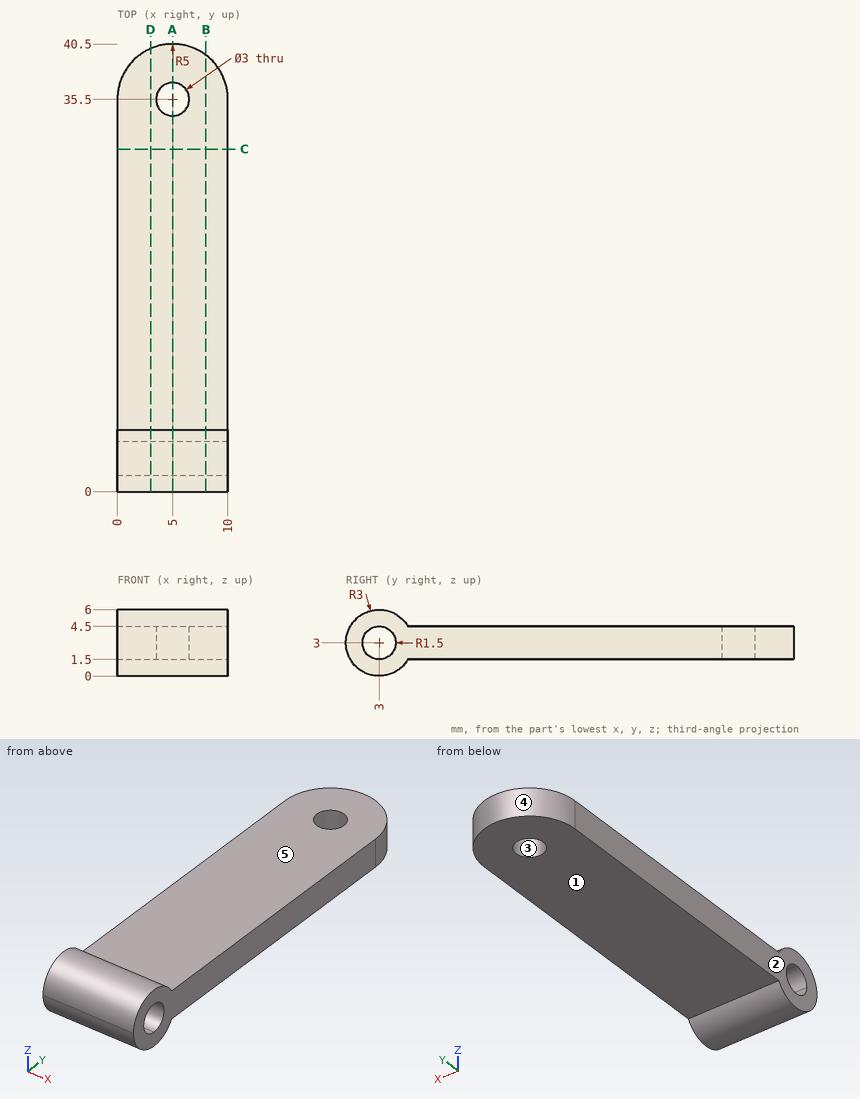
Geometry check sheet. Reference: drawing and pictorial views, mm from the part's lowest x, y, z. A direction names the side the tool comes from. Coordinates: 2 decimals unless noted, no trailing zeros. Write each loop counter-clockwise with the first axis right and the second up, starting at its lowest first coordinate (ties: lowest second). Pieces come first, ordered by that corner, then holes. Notation, with made-up numbers: (61.5, 34.25) -> (88.5, 34.25) arc R24 cw to (88.5, 66.25) -> close; hole circle Ø5 at (28, 37). An arc over 180 degrees is marked (long way). Use a Markdown table: item, result.
1. Tool access check on the marked faces 1 and 2. Record the directions out of +Z, -Z, +X, -X, +Y, -Y that give a thin tool (end or side, any length) a straight path to the whole face; none if there is none.
Reported:
| item | result |
|---|---|
| face 1 | -Z, +X, -X, +Y |
| face 2 | +Z, -Z, -X, +Y, -Y |
2. Sectioned sample at A-A (x = 5). Enter the section's corners in (y, z), plus the area to 3 significant figures.
Reported:
| item | result |
|---|---|
| outline | (5.6, 1.5) -> (34, 1.5) -> (34, 4.5) -> (5.6, 4.5) arc R3 ccw (long way) to start; (37, 1.5) -> (40.5, 1.5) -> (40.5, 4.5) -> (37, 4.5) -> close; hole circle Ø3 at (3, 3) |
| area | 116 mm2 |
3. Sectioned sample at D-D (x = 3). Enter the section's corners in (y, z), plus the area to 3 significant figures.
Reported:
| item | result |
|---|---|
| outline | (5.6, 1.5) -> (40.08, 1.5) -> (40.08, 4.5) -> (5.6, 4.5) arc R3 ccw (long way) to start; hole circle Ø3 at (3, 3) |
| area | 124 mm2 |
4. Scan lines: line 1 along Y through (x, z) = (5, 3.05); line 2 along Y through (x, z) = (4.5, 4); line 3 along Z through (x, y) = (7, 16). Record each from-to range of solid material in increasing order.
Reported:
| item | result |
|---|---|
| line 1 | y = 0 to 1.5, 4.5 to 34, 37 to 40.5 |
| line 2 | y = 0.17 to 1.88, 4.12 to 34.09, 36.91 to 40.47 |
| line 3 | z = 1.5 to 4.5 |
5. Sectioned sample at C-C (y = 31). Enter the section's corners in (x, z), plus the area to 3 significant figures.
Reported:
| item | result |
|---|---|
| outline | (0, 1.5) -> (10, 1.5) -> (10, 4.5) -> (0, 4.5) -> close |
| area | 30.0 mm2 |
6. Sectioned sample at B-B (x = 8). Enter the section's corners in (y, z).
Reported:
| item | result |
|---|---|
| outline | (5.6, 1.5) -> (39.5, 1.5) -> (39.5, 4.5) -> (5.6, 4.5) arc R3 ccw (long way) to start; hole circle Ø3 at (3, 3) |
7. Go/stop test with flat-tipped pins: pin 1 Ø5 at (x, y) = (6, 28) entering from +Z; pin 2 Ø3.5 at (x, y) = (5, 35.5) entering from -Z. Record where each tip stops, or that it passes through.
Reported:
| item | result |
|---|---|
| pin 1 | stops at z = 4.5 |
| pin 2 | stops at z = 1.5 |
8. Release check for a two-part mould opening along X. For the marked faces 3, 4 and 5 record: pulls with the +X half, pulls with the -X half, needs draft (parallel to the pull), parting line crosses it, or undercut.
Reported:
| item | result |
|---|---|
| face 3 | undercut |
| face 4 | parting line crosses it |
| face 5 | needs draft |
